Autodesk Inventor part; units mm, degrees
ref_plane "YZ Plane" through (0, 0, 0) normal (1, 0, 0) x (0, 1, 0)
ref_plane "XZ Plane" through (0, 0, 0) normal (0, 1, 0) x (-1, 0, 0)
ref_plane "XY Plane" through (0, 0, 0) normal (0, 0, 1) x (1, 0, 0)
sketch "Sketch1" plane through (0, 0, 0) normal (0, 0, 1) x (1, 0, 0)
  line L0 (-60, 0) -> (-60, 70)
  line L1 (-60, 70) -> (10, 70)
  line L2 (10, 70) -> (50.9576, 41.3212)
  line L3 (50.9576, 41.3212) -> (50.9576, 0)
  line L4 (53.9576, 0) -> (53.9576, 42.8829)
  line L5 (53.9576, 42.8829) -> (10.9459, 73)
  line L6 (10.9459, 73) -> (-63, 73)
  line L7 (-63, 73) -> (-63, 0)
  line L8 (53.9576, 0) -> (50.9576, 0)
  line L9 (-60, 0) -> (-63, 0)
  point P0 (0, 0)
  dimension "d0" = 70
  dimension "d1" = 70
  dimension "d2" = 145
  dimension "d4" = 50
  dimension "d5" = 60
  dimension "d90" = 3
extrude "Extrusion1" add sketch "Sketch1" along normal blind 200
sketch "Sketch2" plane through (-63, 73, 0) normal (0, 1, 0) x (1, 0, 0)
  line L0 (10, -39.5) -> (56, -39.5)
  line L1 (56, -39.5) -> (56, -85.5)
  line L2 (56, -85.5) -> (10, -85.5)
  line L3 (10, -85.5) -> (10, -39.5)
  line L4 (0, 0) -> (0, -200)
  line L5 (73.9459, 0) -> (0, 0)
  line L6 (56, -160.5) -> (10, -160.5)
  line L7 (56, -114.5) -> (56, -160.5)
  line L8 (10, -160.5) -> (10, -114.5)
  line L9 (10, -114.5) -> (56, -114.5)
  point P0 (63, 0)
  dimension "d9" = 46
  dimension "d10" = 46
  dimension "d11" = 10
  dimension "d12" = 39.5
  dimension "d15" = 75
extrude "Extrusion2" cut sketch "Sketch2" against normal blind 200
sketch "Sketch10" plane through (-63, 0, 0) normal (-1, 0, 0) x (0, 0, 1)
  line L0 (80, 27.5) -> (95, 27.5)
  line L1 (95, 27.5) -> (95, 17.5)
  line L2 (95, 17.5) -> (80, 17.5)
  line L3 (80, 17.5) -> (80, 27.5)
  line L4 (0, 0) -> (200, 0)
  line L5 (0, 73) -> (0, 0)
  dimension "d84" = 17.5
  dimension "d85" = 80
  dimension "d86" = 15
  dimension "d87" = 10
extrude "Extrusion10" cut sketch "Sketch10" against normal blind 10
sketch "Sketch15" plane through (0, 0, 200) normal (0, 0, 1) x (1, 0, 0)
  line L0 (-60, 0) -> (-60, 70)
  line L1 (-60, 0) -> (-60, 70)
  line L2 (10, 70) -> (50.9576, 41.3212)
  line L3 (-60, 70) -> (10, 70)
  line L4 (50.9576, 41.3212) -> (50.9576, 0)
  line L5 (10, 70) -> (50.9576, 41.3212)
  line L6 (50.9576, 41.3212) -> (50.9576, 0)
  line L7 (50.9576, 0) -> (-60, 0)
  point P0 (0, 0)
extrude "Extrusion11" add sketch "Sketch15" against normal blind 3
pattern_linear "Rectangular Pattern3" count 2 spacing 197 along (0, 0, -1) of "Extrusion11"
sketch "Sketch16" plane through (10.9459, 73, 200) normal (0.5736, 0.8192, 0) x (0.8192, -0.5736, 0)
  line L0 (17.5076, 92.5) -> (37.5076, 92.5)
  line L1 (37.5076, 92.5) -> (37.5076, 120)
  line L2 (37.5076, 120) -> (17.5076, 120)
  line L3 (17.5076, 120) -> (17.5076, 92.5)
  line L4 (52.5076, 200) -> (52.5076, 0)
  line L5 (52.5076, 200) -> (0, 200)
  line L6 (18.5076, 151) -> (37.5076, 151)
  line L7 (37.5076, 151) -> (37.5076, 175)
  line L8 (37.5076, 175) -> (18.5076, 175)
  line L9 (18.5076, 175) -> (18.5076, 151)
  circle A0 centre (27.5076, 50) radius 3.25
  line L10 (23.5076, 20) -> (32.5076, 20)
  line L11 (32.5076, 20) -> (32.5076, 29)
  line L12 (32.5076, 29) -> (23.5076, 29)
  line L13 (23.5076, 29) -> (23.5076, 20)
  line L14 (52.5076, 0) -> (0, 0)
  line L15 (7.5, 20) -> (14, 20)
  line L16 (14, 20) -> (14, 71)
  line L17 (14, 71) -> (7.5, 71)
  line L18 (7.5, 71) -> (7.5, 20)
  line L19 (0, 200) -> (0, 0)
  point P0 (32.9047, 200)
  dimension "d99" = 20
  dimension "d100" = 27.5
  dimension "d101" = 15
  dimension "d102" = 80
  dimension "d103" = 24
  dimension "d104" = 19
  dimension "d105" = 15
  dimension "d106" = 25
  dimension "d107" = 6.5
  dimension "d108" = 9
  dimension "d109" = 9
  dimension "d110" = 20
  dimension "d111" = 25
  dimension "d112" = 50
  dimension "d113" = 20
  dimension "d114" = 6.5
  dimension "d115" = 51
  dimension "d116" = 7.5
  dimension "d117" = 20
extrude "Extrusion12" cut sketch "Sketch16" against normal blind 3 contours L3 L2 L1 L0 | L9 L8 L7 L6 | A0 | L13 L12 L11 L10 | L18 L17 L16 L15
sketch "Sketch17" plane through (50.9576, 41.3212, 3) normal (-0.5736, -0.8192, 0) x (0.8192, -0.5736, 0)
  line L0 (-38.4383, 76.75) -> (-8.4383, 76.75)
  line L1 (-8.4383, 76.75) -> (-8.4383, 104.75)
  line L2 (-8.4383, 104.75) -> (-38.4383, 104.75)
  line L3 (-38.4383, 104.75) -> (-38.4383, 76.75)
  line L4 (-46.1959, 118.5) -> (-34.1959, 118.5)
  line L5 (-34.1959, 118.5) -> (-34.1959, 184.5)
  line L6 (-34.1959, 184.5) -> (-46.1959, 184.5)
  line L7 (-46.1959, 184.5) -> (-46.1959, 118.5)
  line L8 (-29.4383, 166) -> (-16.4383, 166)
  line L9 (-16.4383, 166) -> (-16.4383, 179)
  line L10 (-16.4383, 179) -> (-29.4383, 179)
  line L11 (-29.4383, 179) -> (-29.4383, 166)
  line L12 (-36.9459, 177) -> (-36.9459, 126)
  line L13 (-43.4459, 177) -> (-36.9459, 177)
  line L14 (-27.4383, 177) -> (-18.4383, 177)
  line L15 (-27.4383, 168) -> (-27.4383, 177)
  line L16 (-33.4383, 104.5) -> (-13.4383, 104.5)
  line L17 (-33.4383, 77) -> (-33.4383, 104.5)
  line L18 (-35.4383, 21) -> (-10.4383, 21)
  line L19 (-10.4383, 21) -> (-10.4383, 47)
  line L20 (-10.4383, 47) -> (-35.4383, 47)
  line L21 (-35.4383, 47) -> (-35.4383, 21)
  line L22 (-32.4383, 46) -> (-13.4383, 46)
  line L23 (-32.4383, 22) -> (-32.4383, 46)
  point P0 (-18.0412, -3)
  point P1 (-34.1959, 151.5)
  point P2 (-36.9459, 151.5)
  point P3 (-40.1959, 177)
  point P4 (-40.1959, 184.5)
  point P5 (-22.9383, 179)
  point P6 (-22.9383, 177)
  point P7 (-29.4383, 172.5)
  point P8 (-27.4383, 172.5)
  point P9 (-23.4383, 104.75)
  point P10 (-23.4383, 104.5)
  point P11 (-33.4383, 90.75)
  point P12 (-38.4383, 90.75)
  point P13 (-22.9383, 47)
  point P14 (-22.9383, 46)
  point P15 (-32.4383, 34)
  point P16 (-35.4383, 34)
  dimension "d120" = 66
  dimension "d121" = 12
  dimension "d122" = 13
  dimension "d123" = 13
  dimension "d124" = 30
  dimension "d125" = 28
  dimension "d126" = 26
  dimension "d127" = 25
extrude "Extrusion13" cut sketch "Sketch17" against normal blind 1.5
properties part number "albox"
The listing builds one solid part. Answer for the finished solid, in the listing's coordinates (mm). A direction names the side the tool comes from. Give positions to 0.01 mm unless a question says otherwise; leave off trailing zeros. Loops run counter-clockwise (first coordinate to the right, second up) from the corner with the lowest first, then second, coordinate; pieces in that order, holes last.
Item 1: Find the intervals of material crossed by line 1 along Z through (x, y) = (-9, 65.5); line 2 along X through (y, z) = (15.5, 15); line 3 along Z through (x, y) = (31, 57), in increasing order.
Derived:
line 1: z = 0 to 3, 197 to 200
line 2: x = -63 to -60, 50.96 to 53.96
line 3: z = 0 to 24, 50 to 79.75, 107.75 to 147.37, 152.63 to 169, 182 to 200
Item 2: A cutting plane is placed at C-C (z = 105). Give the vertices of the cut face in (x, y), then the cut area to 3 significant figures.
Derived:
outline: (-63, 0) - (-60, 0) - (-60, 70) - (10, 70) - (19.47, 63.37) - (20.33, 64.6) - (24.43, 61.73) - (25.29, 62.96) - (10.95, 73) - (-63, 73) - close; (40.81, 50.26) - (44.91, 47.39) - (44.05, 46.16) - (50.96, 41.32) - (50.96, 0) - (53.96, 0) - (53.96, 42.88) - (41.67, 51.49) - close
area: 635 mm2
Item 3: A cutting plane is placed at A-A (z = 52.5). Give the vertices of the cut face in (x, y), then the cut area to 3 significant figures.
Derived:
outline: (-63, 0) - (-60, 0) - (-60, 70) - (-53, 70) - (-53, 73) - (-63, 73) - close; (-7, 70) - (10, 70) - (50.96, 41.32) - (50.96, 0) - (53.96, 0) - (53.96, 42.88) - (10.95, 73) - (-7, 73) - close
area: 572 mm2
Item 4: A tool of negligible diameter and unlimited length cuts with its end or side. For faces 3 (the flat face through (-5, 35, 3)), 4 (the flat face through (22.1, 63.36, 154.96)), 5 (the flat face through (-61, 0, 100)), from which of +Z, -Z, +X, -X, +Y, -Y can it reach the whole face along a straight path? Write none if from no direction.
Derived:
face 3: -Y
face 4: none
face 5: +Z, -Z, +X, -X, -Y
Item 5: A cutting plane is placed at B-B (y = 31). Give the vertices of the cut face in (x, z), then the cut area to 3 significant figures.
Derived:
outline: (-63, 0) - (53.96, 0) - (53.96, 200) - (-63, 200) - close; hole (-60, 3) - (50.96, 3) - (50.96, 197) - (-60, 197) - close
area: 1,870 mm2
Item 6: Each of these flat-tipped pins is pushed along its axis until it touches: pin 1 Ø0.9 at (y, z) = (71.5, 130.5) entering from +X; pin 2 Ø3.5 at (y, z) = (72, 72.5) entering from +X. Where does it stop, or does it pass through?
Derived:
pin 1: stops at x = 13.73
pin 2: stops at x = 14.87
Item 7: Determine the mould class of faces 1 (the flat face through (-26, 73, 99)), 2 (the flat face through (50.958, 21, 99)) for opening direction Z: +Z half, -Z half, draft (parallel to the pull), parting line (faces both ways), or undercut.
Derived:
face 1: draft
face 2: undercut
Item 8: A cutting plane is placed at D-D (x = -55). Give the vertices of the cut face in (y, z).
Derived:
outline: (0, 0) - (73, 0) - (73, 200) - (0, 200) - (0, 197) - (70, 197) - (70, 3) - (0, 3) - close
